from build123d import *

# Parameters (mm, degrees)
F0_R     = 12
F1_DEPTH = 18.5
F0_W     = 10.1
F0_H     = 10.1
F2_DEPTH = 12
F3_SIZE2 = 11.99999
F3_SIZE  = 1.99999
F4_R     = 1
F5_R     = 0.7
F6_R     = 50
F7_SIZE  = 0.8


# Not quite as in the source:
# - a fillet or chamfer is up to 0.001 mm smaller than in the source, because OpenCascade refuses the exact size


with BuildPart() as f1:
    # F0 (on Top) → F1 (new body)
    with BuildSketch(Plane.XY):
        Circle(F0_R)
        Polygon((0, 9.237604307), (8, 4.6188021535), (8, -4.6188021535), (0, -9.237604307), (-8, -4.6188021535), (-8, 4.6188021535), align=None, mode=Mode.SUBTRACT)
    extrude(amount=F1_DEPTH)

    # F0 (on Top) → F2 (join)
    with BuildSketch(Plane.XY):
        Circle(F0_R)
        Polygon((0, 9.237604307), (8, 4.6188021535), (8, -4.6188021535), (0, -9.237604307), (-8, -4.6188021535), (-8, 4.6188021535), align=None, mode=Mode.SUBTRACT)
        Polygon((8, -4.6188021535), (8, 4.6188021535), (0, 9.237604307), (-8, 4.6188021535), (-8, -4.6188021535), (0, -9.237604307), align=None)
        Rectangle(F0_W, F0_H, mode=Mode.SUBTRACT)
    extrude(amount=-F2_DEPTH)

    # F3 (size 2 and 12 in the source; OpenCascade refuses exactly that, so slightly less here)
    f3_edges = [f1.edges().sort_by_distance(p)[0] for p in [
        (-12, 0, -12),
    ]]
    f3_side = f1.faces().sort_by_distance((5.389411, 0, -12))[0]
    chamfer(f3_edges, length=F3_SIZE, length2=F3_SIZE2, reference=f3_side)

    # F4
    f4_edges = [f1.edges().sort_by_distance(p)[0] for p in [
        (-5.05, 5.05, -6),
        (5.05, 5.05, -6),
        (5.05, -5.05, -6),
        (-5.05, -5.05, -6),
    ]]
    fillet(f4_edges, radius=F4_R)

    # F5
    f5_edges = [f1.edges().sort_by_distance(p)[0] for p in [
        (4, -6.928203, 0),
        (-4, -6.928203, 0),
        (5.05, 0, 0),
        (4.757107, 4.757107, 0),
        (4.757107, -4.757107, 0),
        (0, 5.05, 0),
        (0, -5.05, 0),
        (-4.757107, 4.757107, 0),
        (-4.757107, -4.757107, 0),
        (-5.05, 0, 0),
        (-4, 6.928203, 0),
        (4, 6.928203, 0),
        (8, 0, 0),
        (-8, 0, 0),
    ]]
    fillet(f5_edges, radius=F5_R)

    # F6
    f6_edges = [f1.edges().sort_by_distance(p)[0] for p in [
        (-12, 0, -1e-05),
        (-12, 0, 0),
    ]]
    fillet(f6_edges, radius=F6_R)

    # F7
    f7_edges = [f1.edges().sort_by_distance(p)[0] for p in [
        (5.05, 0, -12),
    ]]
    chamfer(f7_edges, length=F7_SIZE)


solid = f1.part
Can you work these out from the model? Positions are in its coordinate system, mm. A direction names the side the tool comes from. Coordinates: 2 decimals unless noted, no trailing zeros. Write each loop counter-clockwise with the first axis right and the second up, starting at its lowest first coordinate (ties: lowest second). Pieces come first, ordered by that corner, then holes. Notation, with made-up numbers: (10.5, 29.25) -> (39.5, 29.25) arc R28 ccw to (39.5, 66.25) -> close; hole circle Ø6 at (-26.5, 41.5). An arc over 180 degrees is marked (long way). Write each question's results on one line, items separated by ' | '. Start each with the question number.
Item 1: If we section it at A-A, the plane z = 13.5: Write out the boundary of the cut face in (x, y), and give its area (3 significant figures).
Item 2: Thinking about a two-plate mould opening in Y: for faces 4 (the flat face through (-3, -8, 18.5)), 5 (the flat face through (0, -5.05, -6)), 6 (the cylindrical face through (11.446, 3.604, 11.42)), 7 (the flat face through (-3.944, -6.961, 9.475)), which applies, released by +Y, released by -Y, zero draft, split by the parting line, or undercut?
Item 3: Please list where these lines run through material, in increasing order: probe 1 along Z at (x, y) = (0.5, -6); probe 2 along X at (y, z) = (2, -9); probe 3 along Y at (x, z) = (-4.25, 17.5).
Item 4: I'm going to push flat-ended pins straight in: P1, Ø6, axis at y = -7.5, z = 3.5, coming from the +X side; P2, Ø4, axis at y = -3.5, z = -0.5, coming from the +X side; P3, Ø12, axis at x = 9, z = -8.5, coming from the -Y side (3 decimals). Where does each tip first touch, or does it pass through?
Item 5: On a 3-axis mill with a long thin cutter (end or side, diameter ignored), from which of +Z, -Z, +X, -X, +Y, -Y can I reach the whole of each face in a straight line? I mean faces 1 (the flat face through (-5.44, 0.06, -11.59)), 2 (the flat face through (5.05, 0, -6)), 3 (the flat face through (0, -6, 0)). Say none if no direction works.
Answer block:
1) outline: circle Ø24 at (0, 0); hole (-8, -4.62) -> (0, -9.24) -> (8, -4.62) -> (8, 4.62) -> (0, 9.24) -> (-8, 4.62) -> close | area: 231 mm²
2) face 4: zero draft | face 5: undercut | face 6: split by the parting line | face 7: undercut
3) probe 1: -12 to 0 | probe 2: -10.31 to -5.05, 5.05 to 10.31 | probe 3: -11.22 to -6.78, 6.78 to 11.22
4) P1: x = 11.12 | P2: x = 11.74 | P3: y = -10.415
5) face 1: -Z | face 2: +Z, -Z | face 3: +Z
